```python
from build123d import *

# Parameters (mm, degrees)
SKETCH1_R           = 3
BOSS_EXTRUDE1_DEPTH = 4
FILLET1_R           = 0.4


with BuildPart() as part:
    # Sketch1 → Boss-Extrude1 (new body)
    with BuildSketch(Plane(origin=(0, 0, 0), x_dir=(1, 0, 0), z_dir=(0, 1, 0))):
        Polygon((0, 6.92820323), (-6, 3.464101615), (-6, -3.464101615), (0, -6.92820323), (6, -3.464101615), (6, 3.464101615), align=None)
        with Locations(Location((0, 0, 0), (0, 0, 270))):
            Circle(SKETCH1_R, mode=Mode.SUBTRACT)
    extrude(amount=BOSS_EXTRUDE1_DEPTH)

    # Fillet1
    fillet1_edges = [part.edges().sort_by_distance(p)[0] for p in [
        (-6, 4, 0),
        (-3, 4, 5.196152423),
        (3, 4, 5.196152423),
        (6, 4, 0),
        (3, 4, -5.196152423),
        (6, 0, 0),
        (3, 0, 5.196152423),
        (-3, 0, 5.196152423),
        (-6, 0, 0),
        (-3, 0, -5.196152423),
        (3, 0, -5.196152423),
        (-3, 4, -5.196152423),
    ]]
    fillet(fillet1_edges, radius=FILLET1_R)


solid = part.part
```
The listing builds one solid part. Answer for the finished solid, in the listing's coordinates (mm). Give positions to 0.01 mm unless a question says otherwise; leave off trailing zeros. Loops run counter-clockwise (first coordinate to the right, second up) from the corner with the lowest first, then second, coordinate; pieces in that order, holes last. Notation, with made-up numbers: (62, 12) - (83, 12) arc R14 cw to (83, 29) - close; hole circle Ø5 at (-28.75, 39.25). An arc over 180 degrees is marked (long way). Return JSON: item names as keys, results as strings. Group by question number.
1. Find section A-A (z = 0). Write down the section's boundary in (x, y), then the cut area to 3 significant figures.
2. Find section B-B (y = 3.35). Write down the section's boundary in (x, z), then the cut area to 3 significant figures.
3. Given pin 1 Ø1 at (x, y) = (3, 3) entering from +Z, flat-ended and moving along its own axis, determine where the tip first touches the part or whether it passes through.
4. Find section C-C (z = -1.5). Write down the section's boundary in (x, y).
5. Straight lines are drawn through the part: line 1 (X direction, y = 2.65, z = 0); line 2 (Z direction, x = 2.5, y = 2.15); line 3 (X direction, y = 1.9, z = -2). For each, find the intervals that lie inside material, in ascending order. Write a range as [from, to].
6. Determine the mould class of faces 1 (the cylindrical face through (0.9, 1.97, 2.86)), 2 (the cylindrical face through (-2.985, 3.88, -5.073)), 3 (the cylindrical face through (2.985, 0.12, 5.073)), 4 (the flat face through (1, 4, 3)) for opening direction Z: pulls with the +Z half, pulls with the -Z half, needs draft (parallel to the pull), parting line crosses it, or undercut.
Verdict:
{
 "1": {"outline": "(-6, 0.4) arc R0.4 ccw to (-5.6, 0) - (-3, 0) - (-3, 4) - (-5.6, 4) arc R0.4 ccw to (-6, 3.6) - close; (3, 0) - (5.6, 0) arc R0.4 ccw to (6, 0.4) - (6, 3.6) arc R0.4 ccw to (5.6, 4) - (3, 4) - close", "area": "23.9 mm^2"},
 "2": {"outline": "(-6, -3.46) - (0, -6.93) - (6, -3.46) - (6, 3.46) - (0, 6.93) - (-6, 3.46) - close; hole circle Ø6 at (0, 0)", "area": "96.4 mm^2"},
 "3": {"pin 1": "stops at z = 5.48"},
 "4": {"outline": "(-6, 0.4) arc R0.4 ccw to (-5.6, 0) - (-2.6, 0) - (-2.6, 4) - (-5.6, 4) arc R0.4 ccw to (-6, 3.6) - close; (2.6, 0) - (5.6, 0) arc R0.4 ccw to (6, 0.4) - (6, 3.6) arc R0.4 ccw to (5.6, 4) - (2.6, 4) - close"},
 "5": {"line 1": "x = [-6, -3], [3, 6]", "line 2": "z = [-5.48, -1.66], [1.66, 5.48]", "line 3": "x = [-6, -2.24], [2.24, 6]"},
 "6": {"face 1": "undercut", "face 2": "pulls with the -Z half", "face 3": "pulls with the +Z half", "face 4": "needs draft"}
}
